Read the model definition and answer for the solid it produces. Units are mm, in the model's axes. A direction names the side the tool comes from. Give positions to 0.01 mm unless a question says otherwise; leave off trailing zeros. Loops run counter-clockwise (first coordinate to the right, second up) from the corner with the lowest first, then second, coordinate; pieces in that order, holes last. Notation, with made-up numbers: (-20, 38.5) - (-12, 38.5) arc R19 ccw to (-12, 44.5) - close; hole circle Ø2 at (-23.5, -18). An arc over 180 degrees is marked (long way). Write each question's results on one line, items separated by ' | '. Start each with the question number.
Q1. Find the intervals of material crossed by line 1 (Y direction, x = 52, z = 0); line 2 (Z direction, x = 47, y = -7); line 3 (Y direction, x = 55.5, z = -7), in increasing order. Write a range as from..to.
Q2. The part is cut by section C-C, the plane z = 14. Write down the section's boundary in (x, y).
Q3. For faces 4 (the flat face through (30, 14.9, -9.5)), 5 (the cylindrical face through (49.07, 6.84, -12.23)), 6 (the flat face through (-3, 12, 0)), 7 (the flat face through (70, 2.7, -7)), determine the directions among +Z, -Z, +X, -X, +Y, -Y from which every point of the face is accessible in a straight line to the end or side of a thin tool.
Q4. The part is cut by section D-D, the plane x = 27. Write down the section's boundary in (y, z).
Q5. Determine the mould class of faces 1 (the flat face through (53, 0, 2)), 2 (the flat face through (-3, -13, 0)), 3 (the cylindrical face through (42.2, 11.2, -14.6)) for opening direction Z: +Z half, -Z half, draft (parallel to the pull), parting line (faces both ways), or undercut.
Q6. Given pin 1 (1 mm diameter, centred on y = 1, z = 4.5, fed in from +X); pin 2 (3 mm diameter, centred on x = 27.5, z = -11.5, fed in from -Y); pin 3 (0.9 mm diameter, centred on y = -15, z = 0, fed in from +X), each flat-ended and moving along its own axis, determine where each tip first touches the part or whether it passes through.
Q7. The part is cut by section A-A, the plane x = 45.5. Write down the section's boundary in (y, z).
Q8. The part is cut by section B-B, the plane y = 0. Write down the section's boundary in (x, z).
```python
from build123d import *

# Parameters (mm, degrees)
ESQUISSE2_R             = 1.5
ENL_V_MAT_EXTRU_1_DEPTH = 10
ENL_V_MAT_EXTRU_2_DEPTH = 1
BOSS_EXTRU_2_DEPTH      = 2
BOSS_EXTRU_2_DEPTH_BACK = 2
ESQUISSE7_W             = 5.6
ESQUISSE7_H             = 1
ESQUISSE9_OUTSIDE_W     = 58.156
ESQUISSE9_OUTSIDE_H     = 58.156
ENL_V_MAT_EXTRU_3_DEPTH = 12


with BuildPart() as part:
    # Esquisse1 → R_volution1 (revolve)
    with BuildSketch(Plane.XY, mode=Mode.PRIVATE) as r_volution1_sk:
        Polygon((30, 17.5), (30, 18.4), (54, 18.4), (54, 0), (0, 0), (0, 17.5), align=None)
    revolve(r_volution1_sk.sketch.rotate(Axis((0, 0, 0), (1, 0, 0)), 90), axis=Axis((0, 0, 0), (1, 0, 0)))

    # Esquisse2 → Enl_v. mat.-Extru.1 (cut)
    with BuildSketch(Plane(origin=(54, 0, 0), x_dir=(0, 0, -1), z_dir=(1, 0, 0))):
        with Locations((0, 15.5)):
            Circle(ESQUISSE2_R)
        with Locations((13.423393759, 7.75)):
            Circle(ESQUISSE2_R)
        with Locations((13.423393759, -7.75)):
            Circle(ESQUISSE2_R)
        with Locations((0, -15.5)):
            Circle(ESQUISSE2_R)
        with Locations((-13.423393759, -7.75)):
            Circle(ESQUISSE2_R)
        with Locations((-13.423393759, 7.75)):
            Circle(ESQUISSE2_R)
    extrude(amount=-ENL_V_MAT_EXTRU_1_DEPTH, mode=Mode.SUBTRACT)

    # Esquisse5 → R_volution2 (revolve)
    with BuildSketch(Plane(origin=(0, 0, 0), x_dir=(1, 0, 0), z_dir=(0, 1, 0)), mode=Mode.PRIVATE) as r_volution2_sk:
        Polygon((54, 7), (76, 7), (76, 10), (60.5, 10), (60.5, 12), (59.5, 13), (54, 13), align=None)
    revolve(r_volution2_sk.sketch.rotate(Axis((54, 0, -7), (1, 0, 0)), 180), axis=Axis((54, 0, -7), (1, 0, 0)))

    # Esquisse6 → Enl_v. mat.-Extru.2 (cut)
    with BuildSketch(Plane(origin=(54, 0, 0), x_dir=(0, 0, -1), z_dir=(1, 0, 0))):
        with BuildLine():
            ThreePointArc((6.98802926, 9.755380416), (-12, 0), (6.98802926, -9.755380416))
            ThreePointArc((6.98802926, -9.755380416), (7.3591047, -8.690855421), (6.481545758, -7.983182649))
            ThreePointArc((6.481545758, -7.983182649), (-1, 0), (6.481545758, 7.983182649))
            ThreePointArc((6.481545758, 7.983182649), (7.3591047, 8.690855421), (6.98802926, 9.755380416))
        make_face()
    extrude(amount=-ENL_V_MAT_EXTRU_2_DEPTH, mode=Mode.SUBTRACT)

    # Esquisse7 → Boss.-Extru.2 (add, two sides: drawn at the far end of the back side and taken through both)
    with BuildSketch(Plane.XY.offset(-BOSS_EXTRU_2_DEPTH_BACK)):
        with Locations((-2.8, 12.5)):
            Rectangle(ESQUISSE7_W, ESQUISSE7_H)
        with Locations((-2.8, -12.5)):
            Rectangle(ESQUISSE7_W, ESQUISSE7_H)
    extrude(amount=BOSS_EXTRU_2_DEPTH + BOSS_EXTRU_2_DEPTH_BACK)

    # Esquisse8 → R_volution3 (revolve)
    with BuildSketch(Plane.XY):
        with BuildLine():
            Line((0, 0), (-1, 0))
            Line((-1, 0), (-1, 4.2))
            ThreePointArc((-1, 4.2), (-0.765685425, 4.765685425), (-0.2, 5))
            Line((-0.2, 5), (0, 5))
            Line((0, 5), (0, 0))
        make_face()
    revolve(axis=Axis((0, 0, 0), (-1, 0, 0)))

    # Esquisse9 outside → Enl_v. mat.-Extru.3 (cut)
    with BuildSketch(Plane(origin=(76, 0, 0), x_dir=(0, 0, -1), z_dir=(1, 0, 0))):
        Rectangle(ESQUISSE9_OUTSIDE_W, ESQUISSE9_OUTSIDE_H)
        with BuildLine():
            Line((5.692330317, 2.7), (8.307669683, 2.7))
            ThreePointArc((8.307669683, 2.7), (7, -3), (5.692330317, 2.7))
        make_face(mode=Mode.SUBTRACT)
    extrude(amount=-ENL_V_MAT_EXTRU_3_DEPTH, mode=Mode.SUBTRACT)


solid = part.part
```
Check sheet entries:
1) line 1: y = -18.4..-17, -14..14, 17..18.4 | line 2: z = -17.02..-14.72, -12.12..12.12, 14.72..17.02 | line 3: y = -6..6
2) outline: (0, -10.5) - (30, -10.5) - (30, -11.94) - (54, -11.94) - (54, -9.13) - (44, -9.13) - (44, -6.37) - (54, -6.37) - (54, 6.37) - (44, 6.37) - (44, 9.13) - (54, 9.13) - (54, 11.94) - (30, 11.94) - (30, 10.5) - (0, 10.5) - close
3) face 4: -X | face 5: +X | face 6: +Z, -Z, -X | face 7: +Z, -Z, +X, +Y
4) outline: circle Ø35 at (0, 0)
5) face 1: undercut | face 2: draft | face 3: parting line
6) pin 1: stops at x = 53 | pin 2: stops at y = -14.36 | pin 3: stops at x = 44
7) outline: circle Ø36.8 at (0, 0); hole circle Ø3 at (-15.5, 0); hole circle Ø3 at (-7.75, -13.42); hole circle Ø3 at (-7.75, 13.42); hole circle Ø3 at (7.75, -13.42); hole circle Ø3 at (7.75, 13.42); hole circle Ø3 at (15.5, 0)
8) outline: (-1, -4.2) arc R0.8 ccw to (-0.2, -5) - (0, -5) - (0, -17.5) - (30, -17.5) - (30, -18.4) - (54, -18.4) - (54, -13) - (59.5, -13) - (60.5, -12) - (60.5, -10) - (76, -10) - (76, -4) - (60.5, -4) - (60.5, -2) - (59.5, -1) - (54, -1) - (54, 1) - (53, 1) - (53, 12) - (54, 12) - (54, 18.4) - (30, 18.4) - (30, 17.5) - (0, 17.5) - (0, 5) - (-0.2, 5) arc R0.8 ccw to (-1, 4.2) - close
